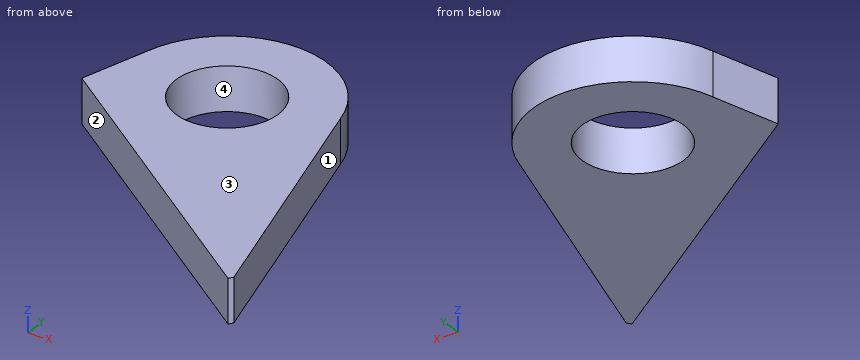
from build123d import *

# Parameters (mm, degrees)
BOSS_EXTRUDE1_DEPTH = 15
SKETCH2_R           = 17.5
CUT_EXTRUDE1_DEPTH  = 87.168439698
CUT_EXTRUDE2_DEPTH  = 15
SKETCH4_W           = 2.2
SKETCH4_H           = 15
CUT_EXTRUDE3_DEPTH  = 10


with BuildPart() as part:
    # Sketch1 → Boss-Extrude1 (new body)
    with BuildSketch(Plane.XY):
        with BuildLine():
            Line((-60, -60), (-33.308172666, 33.308172666))
            ThreePointArc((-33.308172666, 33.308172666), (0, 59.328706637), (33.308172666, 33.308172666))
            Line((33.308172666, 33.308172666), (60, -60))
            Line((60, -60), (-60, -60))
        make_face()
    extrude(amount=BOSS_EXTRUDE1_DEPTH)

    # Sketch2 → Cut-Extrude1 (cut, through all)
    with BuildSketch(Plane.XY.offset(15)):
        with Locations((0, 25)):
            Circle(SKETCH2_R)
    extrude(amount=-CUT_EXTRUDE1_DEPTH, mode=Mode.SUBTRACT)

    # Sketch3 → Cut-Extrude2 (cut)
    with BuildSketch(Plane.XY.offset(15)):
        Polygon((60, -60), (-39.897432064, 10.273715489), (-60, -60), align=None)
    extrude(amount=-CUT_EXTRUDE2_DEPTH, mode=Mode.SUBTRACT)

    # Sketch4 → Cut-Extrude3 (cut)
    with BuildSketch(Plane(origin=(-8.372906684, -11.902485457, 0), x_dir=(0.8179007281921136, -0.5753593649388272, 0), z_dir=(-0.5753593649388272, -0.8179007281921136, 0))):
        with Locations((82.495605588, 7.5)):
            Rectangle(SKETCH4_W, SKETCH4_H)
    extrude(amount=-CUT_EXTRUDE3_DEPTH, mode=Mode.SUBTRACT)


solid = part.part
CAD build for the part. Positions are in the model's coordinates, mm. Face numbers are marked on the shaded views. Round coordinates to 2 decimals unless told otherwise and drop trailing zeros. Write each loop counter-clockwise with the first axis right and the second up, starting at its lowest first coordinate (ties: lowest second). Pieces come first, ordered by that corner, then holes. Notation, with made-up numbers: M -12,-36.5 L 44,-36.5 A20 ccw 44,-31.5 Z; hole C -30.5,68.5 d6. An arc over 180 degrees is marked long. Put each result on its own line as item: value. Start each with the question number.
1) Pull direction Y, two halves, no side cores. Call the marked faces 1, 2, 3 and 4: pulls with the +Y half, pulls with the -Y half, needs draft (parallel to the pull), parting line crosses it, or undercut.
2) Saw through at B-B, the plane z = 6. Write the cut outline in (x, y), and give its area (3 significant figures).
3) Saw through at A-A, the plane x = -12.5. Write the cut outline in (y, z).
4) Saw through at D-D, the plane y = -45.5. Write the cut outline in (x, z), and give its area (3 significant figures).
5) Pin check, flat tips, straight feed: pin 1 Ø3 at (y, z) = (29.5, 9) entering from +X; pin 2 Ø1 at (x, y) = (31.5, 43.5) entering from -Z; pin 3 Ø2 at (x, z) = (-25, 7) entering from +Y; pin 4 Ø8 at (y, z) = (39, 8.5) entering from -X. Stop position of each tip, or through.
6) Drill centre lines: probe 1 along Y at (x, z) = (0, 11); probe 2 along Y at (x, z) = (16, 7.75); probe 3 along X at (y, z) = (13, 2.5). Where is each one in solid material? Low to high. Write a range as [from, to].
7) Saw through at C-C, the plane y = 25. Write the cut outline in (x, z), and give its area (3 significant figures).
Resolved:
1. face 1: pulls with the +Y half
1. face 2: pulls with the -Y half
1. face 3: needs draft
1. face 4: undercut
2. outline: M -39.9,10.27 L 58.2,-58.73 L 59.22,-57.28 L 33.31,33.31 A34.33 ccw -33.31,33.31 Z; hole C 0,25 d35
2. area: 4,810 mm²
3. outline: M -9,0 L 12.75,0 L 12.75,15 L -9,15 Z; M 37.25,0 L 56.97,0 L 56.97,15 L 37.25,15 Z
4. outline: M 39.39,0 L 55.85,0 L 55.85,15 L 39.39,15 Z
4. area: 247 mm²
5. pin 1: x = 34.83
5. pin 2: through
5. pin 3: y = 49.55
5. pin 4: x = -32.84
6. probe 1: [-17.79, 7.5], [42.5, 59.33]
6. probe 2: [-29.05, 17.91], [32.09, 55.37]
6. probe 3: [-39.12, -12.74], [12.74, 39.12]
7. outline: M -35.68,0 L -17.5,0 L -17.5,15 L -35.68,15 Z; M 17.5,0 L 35.68,0 L 35.68,15 L 17.5,15 Z
7. area: 546 mm²
